Design review of the part shown in the three views and the two pictorial views. Dimensions are in mm from the part's minimum x, y and z. A direction names the side the tool comes from. Coordinates: 2 decimals unless noted, no trailing zeros. Order: outer loops, then holes, each group sorted by start corner. A loop starts at its lowest first (then second) coordinate and runs counter-clockwise, first axis right, second up. Notation, with made-up numbers: (-31, 74) -> (-17, 74) arc R7 cw to (-17, 82) -> close; hole circle Ø10 at (55, 81.25). An arc over 180 degrees is marked (long way). Answer as a JSON object with one key per item and string values. Group by question number.
1) Add section A-A, the plane x = 10. Write out the cut boundary in (y, z).
2) Machinability: for the marked faces 1 and 2, which of the approach directions +Z, -Z, +X, -X, +Y, -Y give a long, thin tool a straight path to every point of the face, cutting with its end or side? Answer none if there is none.
3) Add section C-C, the plane x = 34. Write out the cut boundary in (y, z).
4) Add section D-D, the plane z = 17. Write out the cut boundary in (x, y).
5) For pin 1 (3 mm diameter, centred on x = 10, z = 10, fed in from -Y); pin 2 (10 mm diameter, centred on x = 15.5, z = 9, fed in from -Y), all flat-tipped, find the tip position at first contact; note any pin that passes through.
6) Wall thickness on L1, parallel to X at y = 4.9, z = 10; L2, parallel to Z at x = 30, y = 3.6; L3, parallel to Y at x = 22.5, z = 7: over which ranges is each line inside the solid? List them lowest first.
7) Add section B-B, the plane z = 10. Write out the cut boundary in (x, y).
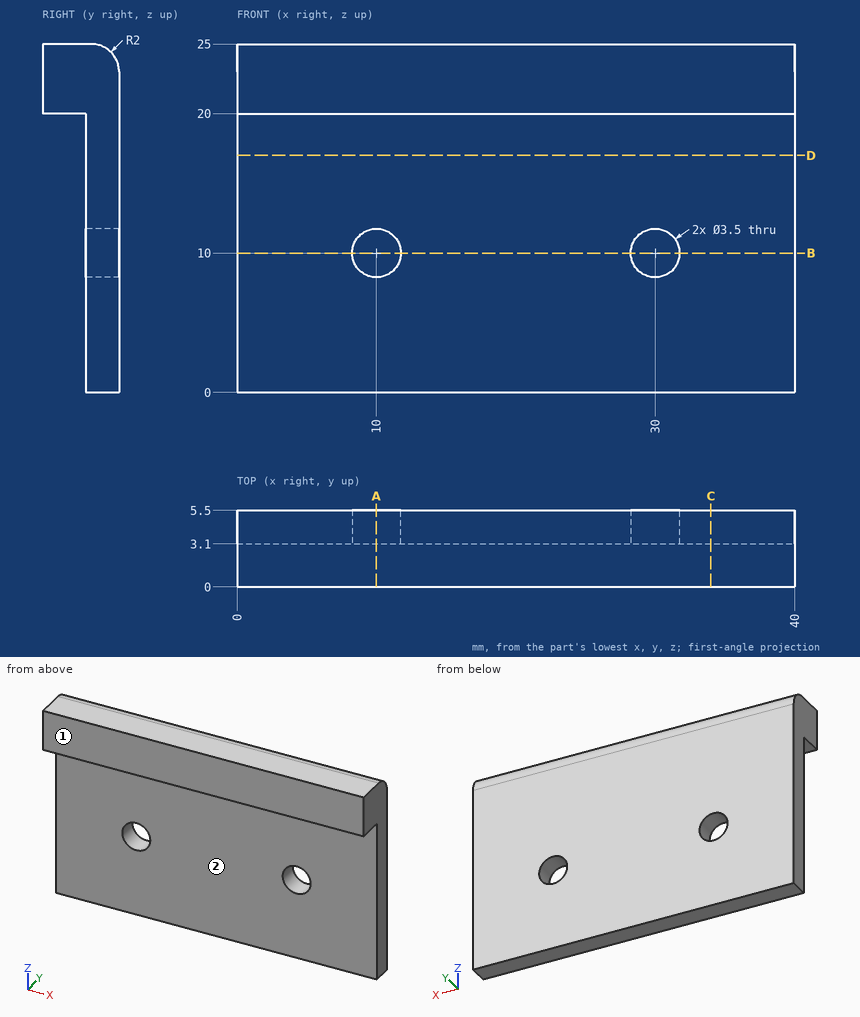
Output values:
{
 "1": {"outline": "(0, 20) -> (3.1, 20) -> (3.1, 11.75) -> (5.5, 11.75) -> (5.5, 23) arc R2 ccw to (3.5, 25) -> (0, 25) -> close; (3.1, 0) -> (5.5, 0) -> (5.5, 8.25) -> (3.1, 8.25) -> close"},
 "2": {"face 1": "+Z, -Z, +X, -X, -Y", "face 2": "-Z, +X, -X, -Y"},
 "3": {"outline": "(0, 20) -> (3.1, 20) -> (3.1, 0) -> (5.5, 0) -> (5.5, 23) arc R2 ccw to (3.5, 25) -> (0, 25) -> close"},
 "4": {"outline": "(0, 3.1) -> (40, 3.1) -> (40, 5.5) -> (0, 5.5) -> close"},
 "5": {"pin 1": "passes through", "pin 2": "stops at y = 3.1"},
 "6": {"L1": "x = 0 to 8.25, 11.75 to 28.25, 31.75 to 40", "L2": "z = 0 to 8.25, 11.75 to 25", "L3": "y = 3.1 to 5.5"},
 "7": {"outline": "(0, 3.1) -> (8.25, 3.1) -> (8.25, 5.5) -> (0, 5.5) -> close; (11.75, 3.1) -> (28.25, 3.1) -> (28.25, 5.5) -> (11.75, 5.5) -> close; (31.75, 3.1) -> (40, 3.1) -> (40, 5.5) -> (31.75, 5.5) -> close"}
}
